CAD build for the part. Positions are in the model's coordinates, mm. A direction names the side the tool comes from. Give positions to 0.01 mm unless a question says otherwise; leave off trailing zeros. Write each loop counter-clockwise with the first axis right and the second up, starting at its lowest first coordinate (ties: lowest second). Pieces come first, ordered by that corner, then holes. Notation, with made-up numbers: (-18.5, 81) -> (27.5, 81) arc R24 cw to (27.5, 113) -> close; hole circle Ø1 at (51, -17). An arc over 180 degrees is marked (long way). Answer in a Markdown table with one row per item. Add a question column.
```python
from build123d import *

# Parameters (mm, degrees)
SKETCH1_W           = 114.3
SKETCH1_H           = 203.2
BOSS_EXTRUDE1_DEPTH = 6.35
SKETCH3_W           = 6.35
SKETCH3_H           = 29.028571428
CUT_EXTRUDE4_DEPTH  = 117.743329574
SKETCH5_W           = 22.86
SKETCH5_H           = 6.35
CUT_EXTRUDE5_DEPTH  = 117.743329574
CUT_EXTRUDE6_DEPTH  = 117.743329574
CAVITY1_START       = -11.43
CAVITY1_OUTLINE_W   = 6.35
CAVITY1_OUTLINE_H   = 6.35
CAVITY1_DEPTH       = 22.86
CAVITY1_START_2     = -50.8
CAVITY1_2_OUTLINE_W = 6.35
CAVITY1_2_OUTLINE_H = 6.35
CAVITY1_2_DEPTH     = 16.51
CAVITY1_START_3     = 34.29
CAVITY1_3_OUTLINE_W = 6.35
CAVITY1_3_OUTLINE_H = 6.35
CAVITY1_3_DEPTH     = 16.51
SKETCH7_R           = 1.4224
CUT_EXTRUDE7_DEPTH  = 117.743329574
SKETCH8_R           = 1.8415
CUT_EXTRUDE8_DEPTH  = 117.743329574


# Read off the part's stored shape, not the designer's step: Cavity1
with BuildPart() as part:
    # Sketch1 → Boss-Extrude1 (new body)
    with BuildSketch(Plane(origin=(0, 0, 0), x_dir=(0, 0, -1), z_dir=(1, 0, 0))):
        Rectangle(SKETCH1_W, SKETCH1_H)
    extrude(amount=BOSS_EXTRUDE1_DEPTH)

    # Sketch3 → Cut-Extrude4 (cut, through all)
    with BuildSketch(Plane(origin=(6.35, 0, 0), x_dir=(0, 0, -1), z_dir=(1, 0, 0))):
        with Locations((-53.975, -58.057142857)):
            Rectangle(SKETCH3_W, SKETCH3_H)
        with Locations((-53.975, 0)):
            Rectangle(SKETCH3_W, SKETCH3_H)
        with Locations((-53.975, 58.057142857)):
            Rectangle(SKETCH3_W, SKETCH3_H)
        with Locations((53.975, 58.057142857)):
            Rectangle(SKETCH3_W, SKETCH3_H)
        with Locations((53.975, 0)):
            Rectangle(SKETCH3_W, SKETCH3_H)
        with Locations((53.975, -58.057142857)):
            Rectangle(SKETCH3_W, SKETCH3_H)
    extrude(amount=-CUT_EXTRUDE4_DEPTH, mode=Mode.SUBTRACT)

    # Sketch5 → Cut-Extrude5 (cut, through all)
    with BuildSketch(Plane(origin=(6.35, 0, 0), x_dir=(0, 0, -1), z_dir=(1, 0, 0))):
        with Locations((-22.86, -98.425)):
            Rectangle(SKETCH5_W, SKETCH5_H)
        with Locations((22.86, -98.425)):
            Rectangle(SKETCH5_W, SKETCH5_H)
    extrude(amount=-CUT_EXTRUDE5_DEPTH, mode=Mode.SUBTRACT)

    # Sketch6 → Cut-Extrude6 (cut, through all)
    with BuildSketch(Plane(origin=(6.35, 0, 0), x_dir=(0, 0, -1), z_dir=(1, 0, 0))):
        Polygon((0, 55.88), (50.8, 55.88), (50.8, 72.571428571), (57.15, 72.571428571), (57.15, 101.6), (-57.15, 101.6), (-57.15, 72.571428571), (-50.8, 72.571428571), (-50.8, 55.88), align=None)
    extrude(amount=-CUT_EXTRUDE6_DEPTH, mode=Mode.SUBTRACT)

    # Cavity1 outline → Cavity1 (cut)
    with BuildSketch(Plane.XY.offset(CAVITY1_START)):
        with Locations((3.175, 52.705)):
            Rectangle(CAVITY1_OUTLINE_W, CAVITY1_OUTLINE_H)
    extrude(amount=CAVITY1_DEPTH, mode=Mode.SUBTRACT)

    # Cavity1 2 outline → Cavity1 2 (cut)
    with BuildSketch(Plane.XY.offset(CAVITY1_START_2)):
        with Locations((3.175, 52.705)):
            Rectangle(CAVITY1_2_OUTLINE_W, CAVITY1_2_OUTLINE_H)
    extrude(amount=CAVITY1_2_DEPTH, mode=Mode.SUBTRACT)

    # Cavity1 3 outline → Cavity1 3 (cut)
    with BuildSketch(Plane.XY.offset(CAVITY1_START_3)):
        with Locations((3.175, 52.705)):
            Rectangle(CAVITY1_3_OUTLINE_W, CAVITY1_3_OUTLINE_H)
    extrude(amount=CAVITY1_3_DEPTH, mode=Mode.SUBTRACT)

    # Sketch7 → Cut-Extrude7 (cut, through all)
    with BuildSketch(Plane(origin=(6.35, 0, 0), x_dir=(0, 0, -1), z_dir=(1, 0, 0))):
        with Locations((18.487090642, 22.207344877)):
            Circle(SKETCH7_R)
        with Locations((21.143949011, -14.574648396)):
            Circle(SKETCH7_R)
    extrude(amount=-CUT_EXTRUDE7_DEPTH, mode=Mode.SUBTRACT)

    # Sketch8 → Cut-Extrude8 (cut, through all)
    with BuildSketch(Plane.ZY):
        with Locations((-35.56, -47.244)):
            Circle(SKETCH8_R)
        with Locations((-8.89, -47.244)):
            Circle(SKETCH8_R)
        with Locations((-35.56, -80.01)):
            Circle(SKETCH8_R)
        with Locations((-8.89, -80.01)):
            Circle(SKETCH8_R)
    extrude(amount=-CUT_EXTRUDE8_DEPTH, mode=Mode.SUBTRACT)


solid = part.part
```
Item 1: Slice it at D-D, the plane z = 7. List the corners of the cut face in (x, y).
Item 2: Slice it at B-B, the plane z = -8.89. List the corners of the cut face in (x, y), then the cut area to 3 significant figures.
Item 3: Slice it at A-A, the plane y = -80.01. List the corners of the cut face in (x, z).
Item 4: Which spindle directions (+Z, -Z, +X, -X, +Y, -Y) get a long thin tool onto all of the face, cutting with end or side? Do faces 1 (the face through (3, 53, 11.43)), 2 (the face through (3, -58, 50.8)), 3 (the face through (3, -58, -50.8)). Say none if no direction does.
Item 5: Probe L1, parallel to Y at x = 5.25, z = -35.56; L2, parallel to Z at x = 2.75, y = -80.01; L3, parallel to Z at x = 2.5, y = 45.5. List the from-to ranges inside material, lowest first. Write a range as from..to.
Item 6: Slice it at C-C, the plane y = 1. List the corners of the cut face in (x, z).
Item 7: Mould opens along Y. For faces 4 (the face through (3, 14.514, -54)), 5 (the face through (3, -95.25, 23)), 6 (the face through (3, -29, -57.15)) say: released by +Y, released by -Y, zero draft, split by the parting line, or undercut.
Item 8: Drop flat-ended pins along their axis: pin 1 Ø3 at (x, z) = (2, -24) entering from -Y; pin 2 Ø3 at (x, y) = (4.5, -4) entering from -Z; pin 3 Ø1.5 at (x, y) = (1, -13) entering from +Z. Give the stop position or say it passes through.
Answer key:
| question | item | result |
|---|---|---|
| 1 | outline | (0, -101.6) -> (6.35, -101.6) -> (6.35, 49.53) -> (0, 49.53) -> close |
| 2 | outline | (0, -101.6) -> (6.35, -101.6) -> (6.35, -81.85) -> (0, -81.85) -> close; (0, -78.17) -> (6.35, -78.17) -> (6.35, -49.09) -> (0, -49.09) -> close; (0, -45.4) -> (6.35, -45.4) -> (6.35, 49.53) -> (0, 49.53) -> close |
| 2 | area | 913 mm² |
| 3 | outline | (0, -57.15) -> (6.35, -57.15) -> (6.35, -37.4) -> (0, -37.4) -> close; (0, -33.72) -> (6.35, -33.72) -> (6.35, -10.73) -> (0, -10.73) -> close; (0, -7.05) -> (6.35, -7.05) -> (6.35, 57.15) -> (0, 57.15) -> close |
| 4 | face 1 | +X, -X, +Y |
| 4 | face 2 | +Z, +X, -X |
| 4 | face 3 | -Z, +X, -X |
| 5 | L1 | y = -101.6..-81.85, -78.17..-49.09, -45.4..49.53 |
| 5 | L2 | z = -57.15..-37.4, -33.72..-10.73, -7.05..57.15 |
| 5 | L3 | z = -50.8..50.8 |
| 6 | outline | (0, -50.8) -> (6.35, -50.8) -> (6.35, 50.8) -> (0, 50.8) -> close |
| 7 | face 4 | undercut |
| 7 | face 5 | released by -Y |
| 7 | face 6 | zero draft |
| 8 | pin 1 | stops at y = -95.25 |
| 8 | pin 2 | stops at z = -50.8 |
| 8 | pin 3 | stops at z = 50.8 |
